Source: CAD feature listing. Evaluate the final solid. Frame: model axes, mm. A direction names the side the tool comes from. Give positions to 0.01 mm unless a question says otherwise; leave off trailing zeros. Loops run counter-clockwise (first coordinate to the right, second up) from the corner with the lowest first, then second, coordinate; pieces in that order, holes last. Notation, with made-up numbers: M 70,-6 L 79,-6 A18 ccw 79,11 Z; hole C -34,68 d3. An arc over 180 degrees is marked long. Put each result on its own line as item: value. Start each with the question number.
```python
from build123d import *

# Parameters (mm, degrees)
SKIZZE2_W                       = 240
SKIZZE2_H                       = 120
SKIZZE2_W_2                     = 10
SKIZZE2_H_2                     = 20
SKIZZE2_W_3                     = 20
SKIZZE2_H_3                     = 5
AUFSATZ_LINEAR_AUSTRAGEN1_DEPTH = 5
SKIZZE3_W                       = 3
SKIZZE3_H                       = 90
SCHNITT_LINEAR_AUSTRAGEN1_DEPTH = 146.430395722
LINEARES_MUSTER1_COUNT          = 9
LINEARES_MUSTER1_PITCH          = 12
SKIZZE4_W                       = 78.5
SKIZZE4_H                       = 20
SCHNITT_LINEAR_AUSTRAGEN2_DEPTH = 146.430395722


with BuildPart() as part:
    # Skizze2 → Aufsatz-Linear austragen1 (new body)
    with BuildSketch(Plane(origin=(0, 0, 0), x_dir=(0, 0, -1), z_dir=(1, 0, 0))):
        Rectangle(SKIZZE2_W, SKIZZE2_H)
        with Locations((-125, 50)):
            Rectangle(SKIZZE2_W_2, SKIZZE2_H_2)
        with Locations((125, 50)):
            Rectangle(SKIZZE2_W_2, SKIZZE2_H_2)
        with Locations((-90, -62.5)):
            Rectangle(SKIZZE2_W_3, SKIZZE2_H_3)
        with Locations((90, -62.5)):
            Rectangle(SKIZZE2_W_3, SKIZZE2_H_3)
    extrude(amount=AUFSATZ_LINEAR_AUSTRAGEN1_DEPTH)

    # Skizze3 → Schnitt-Linear austragen1 (cut, through all)
    with BuildSketch(Plane.ZY):
        Rectangle(SKIZZE3_W, SKIZZE3_H)
    schnitt_linear_austragen1 = extrude(amount=-SCHNITT_LINEAR_AUSTRAGEN1_DEPTH, mode=Mode.SUBTRACT)

    # Lineares Muster1: Schnitt-Linear austragen1 ×9
    with Locations(*[(0, 0, -i * LINEARES_MUSTER1_PITCH) for i in range(1, LINEARES_MUSTER1_COUNT)]):
        add(schnitt_linear_austragen1, mode=Mode.SUBTRACT)

    # Skizze4 → Schnitt-Linear austragen2 (cut, through all)
    with BuildSketch(Plane.ZY):
        with Locations((60.75, 0)):
            Rectangle(SKIZZE4_W, SKIZZE4_H)
        with Locations((60.75, -35)):
            Rectangle(SKIZZE4_W, SKIZZE4_H)
        with Locations((60.75, 35)):
            Rectangle(SKIZZE4_W, SKIZZE4_H)
    extrude(amount=-SCHNITT_LINEAR_AUSTRAGEN2_DEPTH, mode=Mode.SUBTRACT)


solid = part.part
```
1. Section A-A, the plane z = 34.5. Output: boundary loops of the cut face in (x, y), plus the area to 3 significant figures.
2. Pull-direction query (Z, two-part tool) for faces 4 (the face through (2, -60, -110)), 5 (the face through (2, -1, -58.5)), 6 (the face through (2, -63, -100)); classes: released by +Z, released by -Z, zero draft, split by the parting line, or undercut.
3. Ray query, line 1 (Y direction, x = 3.25, z = 83.5); line 2 (Y direction, x = 1.6, z = 57.5); line 3 (Z direction, x = 0.8, y = -52.5). Return the intervals inside material, ascending.
4. Contact query for flat-ended pins moving along their axis: pin 1 (2.5 mm diameter, centred on x = 2.5, z = 1, fed in from -Y); pin 2 (3 mm diameter, centred on x = 2, y = 29.5, fed in from +Z); pin 3 (4 mm diameter, centred on y = -44, z = 32, fed in from -X); pin 4 (1 mm diameter, centred on x = 3, y = 28.5, fed in from -Z). Output: stop coordinate, or through.
5. Section B-B, the plane y = 22.5. State how many separate pieces and enclosed holes the cut face has, plus the area to 4 significant figures.
6. Set-up query: faces 1 (the face through (5, -2, 2)), 2 (the face through (2, -63, -80)), 3 (the face through (2, -1, -49.5)). Return all of +Z, -Z, +X, -X, +Y, -Y with unobstructed straight access to the full face (end or side cutting, diameter ignored); none if empty.
Results found:
1. outline: M 0,-60 L 5,-60 L 5,-45 L 0,-45 Z; M 0,-25 L 5,-25 L 5,-10 L 0,-10 Z; M 0,10 L 5,10 L 5,25 L 0,25 Z; M 0,45 L 5,45 L 5,60 L 0,60 Z
1. area: 300 mm²
2. face 4: zero draft
2. face 5: undercut
2. face 6: released by -Z
3. line 1: -65 to -45, -25 to -10, 10 to 25, 45 to 60
3. line 2: -60 to -45, -25 to -10, 10 to 25, 45 to 60
3. line 3: -120 to 120
4. pin 1: y = -60
4. pin 2: z = 120
4. pin 3: x = 0
4. pin 4: z = -120
5. separate pieces: 10
5. enclosed holes: 0
5. area: 1,065 mm²
6. face 1: +Z, -Z, +X, +Y, -Y
6. face 2: +X, -X, -Y
6. face 3: +X, -X
